For this review, take the finished solid that the model builds, in its own axes (mm). A direction names the side the tool comes from. Coordinates: 2 decimals unless noted, no trailing zeros. Loops run counter-clockwise (first coordinate to the right, second up) from the corner with the lowest first, then second, coordinate; pieces in that order, holes last.
1. To check wall thickness, follow probe 1 along Z at (x, y) = (-0.75, 3.25); probe 2 along X at (y, z) = (-1.75, -122); probe 3 along X at (y, z) = (-2.75, 95). State the ranges of each line that lie inside material, in increasing order.
2. Machinability: for faces 4 (the face through (-1.19, -5.37, -22.02)), 5 (the face through (-3.32, -3.04, -150.57)), 6 (the face through (-5, 0, 66)), 7 (the face through (-6, 0, -11)), which of the approach directions +Z, -Z, +X, -X, +Y, -Y give a long, thin tool a straight path to every point of the face, cutting with its end or side? Answer none if there is none.
3. Mouldability with a two-part tool opening along Z and no side actions: class faces 1 (the face through (-2.5, 3.92, 62.35)), 2 (the face through (0, 0, 134.992)), 3 (the face through (-3.32, -3.04, -163.96)) as pulls with the +Z half, pulls with the -Z half, needs draft (parallel to the pull), parting line crosses it, or undercut.
4. Clearance check with flat-ended pins moving along their axes: P1, Ø4, axis at x = -1, z = 80.5, coming from the -Y side; P2, Ø1.5, axis at x = 0, z = -157, coming from the +Y side; P3, Ø0.9, axis at x = 0.5, z = -49.5, coming from the +Y side. State where each tip first meets the part, or that it passes through.
5. Take a section at A-A, the plane z = 13. State the section outline as (x, y) points.
6. Take a section at B-B, the plane z = -37.5. State the section outline as (x, y) points, then the cut area to 3 significant figures.
```python
from build123d import *

# Parameters (mm, degrees)
SKETCH7_W           = 10
SKETCH7_H           = 1.5
CUT_EXTRUDE4_DEPTH  = 1.5
SKETCH8_W           = 10
SKETCH8_H           = 1.5
CUT_EXTRUDE5_DEPTH  = 1.5
SKETCH11_W          = 1
SKETCH11_H          = 0.35
SKETCH12_W          = 1
SKETCH12_H          = 0.35
SKETCH14_R          = 6
BOSS_EXTRUDE1_DEPTH = 20
BOSS_EXTRUDE2_START = 20
SKETCH15_R          = 6
BOSS_EXTRUDE2_DEPTH = 20
SKETCH18_W          = 1
SKETCH18_H          = 0.35
SKETCH19_W          = 1
SKETCH19_H          = 0.35
SKETCH22_W          = 0.996061345
SKETCH22_H          = 0.5
SKETCH26_W          = 1.000081644
SKETCH26_H          = 0.3
SKETCH27_W          = 1.000526486
SKETCH27_H          = 0.3
SKETCH29_W          = 1
SKETCH29_H          = 0.5
FILLET2_R           = 1
FILLET3_R           = 1
FILLET4_R           = 1
FILLET5_R           = 1
FILLET6_R           = 1
FILLET7_R           = 1


# Some blends are built 0.0001 mm under size
with BuildPart() as part:
    # Sketch1 → Revolve1 (revolve)
    with BuildSketch(Plane(origin=(0, 0, 0), x_dir=(0, 0, -1), z_dir=(1, 0, 0)), mode=Mode.PRIVATE) as revolve1_sk:
        Polygon((-134.992104591, 0), (165.007895409, 0), (165.007895409, 4.5), (149.357384883, 4.5), (149.357384883, 5), (59.357384883, 5), (59.357384883, 6), (19.357384883, 6), (19.357384883, 5), (-134.992104591, 5), align=None)
    revolve(revolve1_sk.sketch.rotate(Axis((0, 0, 134.992104591), (0, 0, -1)), 90), axis=Axis((0, 0, 134.992104591), (0, 0, -1)))

    # Sketch7 → Cut-Extrude4 (cut, symmetric)
    with BuildSketch(Plane(origin=(0, 0, 0), x_dir=(0, 0, -1), z_dir=(1, 0, 0))):
        with Locations((51.512242661, 5.25)):
            Rectangle(SKETCH7_W, SKETCH7_H)
    extrude(amount=CUT_EXTRUDE4_DEPTH, both=True, mode=Mode.SUBTRACT)

    # Sketch8 → Cut-Extrude5 (cut, symmetric)
    with BuildSketch(Plane(origin=(0, 0, 0), x_dir=(0, 0, -1), z_dir=(1, 0, 0))):
        with Locations((156.934482796, 3.75)):
            Rectangle(SKETCH8_W, SKETCH8_H)
    extrude(amount=CUT_EXTRUDE5_DEPTH, both=True, mode=Mode.SUBTRACT)

    # Cut-Sweep1: sweep along a path in Sketch10
    with BuildLine(Plane(origin=(0, 0, -137.647384883), x_dir=(-1, 0, 0), z_dir=(0, 0, -1))) as cut_sweep1_path:
        CenterArc((0, 0), 5, 0, 360)
    # Sketch11 → Cut-Sweep1 (sweep, cut)
    with BuildSketch(Plane(origin=(0, 0, 0), x_dir=(0, 0, -1), z_dir=(1, 0, 0))):
        with Locations((137.649818054, 4.825)):
            Rectangle(SKETCH11_W, SKETCH11_H)
    sweep(path=cut_sweep1_path.line, mode=Mode.SUBTRACT)

    # Cut-Sweep2: sweep along a path in Sketch9
    with BuildLine(Plane(origin=(0, 0, -144.647384883), x_dir=(-1, 0, 0), z_dir=(0, 0, -1))) as cut_sweep2_path:
        CenterArc((0, 0), 5, 0, 360)
    # Sketch12 → Cut-Sweep2 (sweep, cut)
    with BuildSketch(Plane(origin=(0, 0, 0), x_dir=(0, 0, -1), z_dir=(1, 0, 0))):
        with Locations((144.648120844, 4.825)):
            Rectangle(SKETCH12_W, SKETCH12_H)
    sweep(path=cut_sweep2_path.line, mode=Mode.SUBTRACT)

    # Sketch14 → Boss-Extrude1 (add)
    with BuildSketch(Plane(origin=(0, 0, -59.357384883), x_dir=(-1, 0, 0), z_dir=(0, 0, -1))):
        with Locations(Location((0, 0, 0), (0, 0, 180))):
            Circle(SKETCH14_R)
    extrude(amount=BOSS_EXTRUDE1_DEPTH)

    # Sketch15 → Boss-Extrude2 (add)
    with BuildSketch(Plane.XY.offset(-19.357384883).offset(BOSS_EXTRUDE2_START)):
        Circle(SKETCH15_R)
    extrude(amount=-BOSS_EXTRUDE2_DEPTH)

    # Cut-Sweep3: sweep along a path in Sketch16
    with BuildLine(Plane(origin=(0, 0, 62.352615117), x_dir=(-1, 0, 0), z_dir=(0, 0, -1))) as cut_sweep3_path:
        CenterArc((0, 0), 5, 0, 360)
    # Sketch18 → Cut-Sweep3 (sweep, cut)
    with BuildSketch(Plane(origin=(0, 0, 0), x_dir=(0, 0, -1), z_dir=(1, 0, 0))):
        with Locations((-62.354294527, 4.825)):
            Rectangle(SKETCH18_W, SKETCH18_H)
    sweep(path=cut_sweep3_path.line, mode=Mode.SUBTRACT)

    # Cut-Sweep4: sweep along a path in Sketch17
    with BuildLine(Plane(origin=(0, 0, 69.352615117), x_dir=(-1, 0, 0), z_dir=(0, 0, -1))) as cut_sweep4_path:
        CenterArc((0, 0), 5, 0, 360)
    # Sketch19 → Cut-Sweep4 (sweep, cut)
    with BuildSketch(Plane(origin=(0, 0, 0), x_dir=(0, 0, -1), z_dir=(1, 0, 0))):
        with Locations((-69.328460844, 4.825)):
            Rectangle(SKETCH19_W, SKETCH19_H)
    sweep(path=cut_sweep4_path.line, mode=Mode.SUBTRACT)

    # Cut-Sweep5: sweep along a path in Sketch20
    with BuildLine(Plane.XY.offset(-57.012242661)) as cut_sweep5_path:
        CenterArc((0, 0), 6, 0, 360)
    # Sketch22 → Cut-Sweep5 (sweep, cut)
    with BuildSketch(Plane(origin=(0, 0, 0), x_dir=(0, 0, -1), z_dir=(1, 0, 0))):
        with Locations((57.010273334, 5.75)):
            Rectangle(SKETCH22_W, SKETCH22_H)
    sweep(path=cut_sweep5_path.line, mode=Mode.SUBTRACT)

    # Cut-Sweep7: sweep along a path in Sketch24
    with BuildLine(Plane.XY.offset(-162.434482796)) as cut_sweep7_path:
        CenterArc((0, 0), 4.5, 0, 360)
    # Sketch26 → Cut-Sweep7 (sweep, cut)
    with BuildSketch(Plane(origin=(0, 0, 0), x_dir=(0, 0, -1), z_dir=(1, 0, 0))):
        with Locations((162.434523618, 4.35)):
            Rectangle(SKETCH26_W, SKETCH26_H)
    sweep(path=cut_sweep7_path.line, mode=Mode.SUBTRACT)

    # Cut-Sweep8: sweep along a path in Sketch25
    with BuildLine(Plane(origin=(0, 0, -151.434482796), x_dir=(-1, 0, 0), z_dir=(0, 0, -1))) as cut_sweep8_path:
        CenterArc((0, 0), 4.5, 0, 360)
    # Sketch27 → Cut-Sweep8 (sweep, cut)
    with BuildSketch(Plane(origin=(0, 0, 0), x_dir=(0, 0, -1), z_dir=(1, 0, 0))):
        with Locations((151.434219553, 4.35)):
            Rectangle(SKETCH27_W, SKETCH27_H)
    sweep(path=cut_sweep8_path.line, mode=Mode.SUBTRACT)

    # Cut-Sweep9: sweep along a path in Sketch28
    with BuildLine(Plane.XY.offset(-22.012242661)) as cut_sweep9_path:
        CenterArc((0, 0), 6, 0, 360)
    # Sketch29 → Cut-Sweep9 (sweep, cut)
    with BuildSketch(Plane(origin=(0, 0, 0), x_dir=(0, 0, -1), z_dir=(1, 0, 0))):
        with Locations((22.013204975, 5.75)):
            Rectangle(SKETCH29_W, SKETCH29_H)
    sweep(path=cut_sweep9_path.line, mode=Mode.SUBTRACT)

    # Fillet2
    # the kernel refuses this fillet: 1 mm, written as the material it adds along each edge
    with BuildSketch(Plane(origin=(0, 0, -149.357384883), x_dir=(1, 0, 0), z_dir=(0, 1, 0))) as fillet2_piece_1:
        with BuildLine():
            CenterArc((5.5, 0.866025404), FILLET2_R, 180, 60)
            Line((5, 0), (4.99, -0.017320508))
            ThreePointArc((4.99, -0.017320508), (4.75, -0.02), (4.5, -0.02))
            Line((4.5, -0.02), (4.48, 0))
            Line((4.48, 0), (4.48, 0.866025404))
            Line((4.48, 0.866025404), (4.5, 0.866025404))
        make_face()
    revolve(axis=Axis((0, 0, -149.357384883), (0, 0, -1)))

    # Fillet3
    fillet3_edges = [part.edges().sort_by_distance(p)[0] for p in [
        (-5, 0, -149.357384883),
    ]]
    fillet(fillet3_edges, radius=FILLET3_R)

    # Fillet4
    fillet4_edges = [part.edges().sort_by_distance(p)[0] for p in [
        (-6, 0, -79.357384883),
    ]]
    fillet(fillet4_edges, radius=FILLET4_R - 0.0001)  # a hair under: the kernel refuses the full size

    # Fillet5
    fillet5_edges = [part.edges().sort_by_distance(p)[0] for p in [
        (-5, 0, -79.357384883),
    ]]
    fillet(fillet5_edges, radius=FILLET5_R)

    # Fillet6
    fillet6_edges = [part.edges().sort_by_distance(p)[0] for p in [
        (-6, 0, 0.642615117),
    ]]
    fillet(fillet6_edges, radius=FILLET6_R - 0.0001)  # a hair under: the kernel refuses the full size

    # Fillet7
    fillet7_edges = [part.edges().sort_by_distance(p)[0] for p in [
        (-5, 0, 0.642615117),
    ]]
    fillet(fillet7_edges, radius=FILLET7_R)


solid = part.part
```
Results list:
1. probe 1: z = -165.01 to -161.93, -151.93 to 134.99
1. probe 2: x = -4.68 to 4.68
1. probe 3: x = -4.18 to 4.18
2. face 4: none
2. face 5: -Z
2. face 6: +Z
2. face 7: +Z, -Z
3. face 1: undercut
3. face 2: pulls with the +Z half
3. face 3: needs draft
4. P1: stops at y = -5
4. P2: stops at y = 3
4. P3: stops at y = 4.5
5. outline: circle Ø10 at (0, 0)
6. outline: circle Ø12 at (0, 0)
6. area: 113 mm2
